Geometry: final body of the model. Coordinates: model frame, mm. A direction names the side the tool comes from. Coordinates: 2 decimals unless noted, no trailing zeros. Write each loop counter-clockwise with the first axis right and the second up, starting at its lowest first coordinate (ties: lowest second). Pieces come first, ordered by that corner, then holes.
Autodesk Inventor part; units mm, degrees
ref_plane "pc_body_XY" through (6, 12, 0) normal (1, 0, 0) x (0, 0, -1)
ref_plane "pc_body_YZ" through (6, 12, 0) normal (0, 0, -1) x (0, 1, 0)
ref_plane "pc_body_ZX" through (6, 12, 0) normal (0, 1, 0) x (1, 0, 0)
sketch "Sketch_1" plane through (0, 0, 0) normal (1, 0, 0) x (0, 1, 0)
  line L0 (16, 38.5) -> (0.5, 38.5)
  arc A0 (0.5, 38.5) -> (0, 38) centre (0.5, 38) ccw
  line L1 (0, 38) -> (0, 36.5)
  line L2 (0, 36.5) -> (15.75, 36.5)
  line L3 (15.75, 36.5) -> (15.75, 29.5)
  line L4 (15.75, 29.5) -> (12, 29.5)
  line L5 (12, 29.5) -> (12, 18.5)
  line L6 (12, 18.5) -> (15.75, 18.5)
  line L7 (15.75, 18.5) -> (15.75, -18.5)
  line L8 (15.75, -18.5) -> (12, -18.5)
  line L9 (12, -18.5) -> (12, -29.5)
  line L10 (12, -29.5) -> (15.75, -29.5)
  line L11 (15.75, -29.5) -> (15.75, -36.5)
  line L12 (15.75, -36.5) -> (0, -36.5)
  line L13 (0, -36.5) -> (0, -38)
  arc A1 (0, -38) -> (0.5, -38.5) centre (0.5, -38) ccw
  line L14 (0.5, -38.5) -> (16, -38.5)
  arc A2 (16, -38.5) -> (18, -36.5) centre (16, -36.5) ccw
  line L15 (18, -36.5) -> (18, 36.5)
  arc A3 (18, 36.5) -> (16, 38.5) centre (16, 36.5) ccw
extrude "Extrusion1" add sketch "Sketch_1" along normal blind 365
sketch "Sketch_3" plane through (6, 0, 0) normal (1, 0, 0) x (0, 0, -1)
  line L0 (-24, 19.95) -> (-24, 18)
  line L1 (-24, 18) -> (-27.8, 18)
  line L2 (-27.8, 18) -> (-27.8, 19.95)
  line L3 (-27.8, 19.95) -> (-24, 19.95)
  line L4 (-24, 19.95) -> (-24, 18)
revolve "Revolution1" add sketch "Sketch_3" angle 360 about axis through (6, 19.95, 24) along (0, 1, 0)
pattern_linear "Rectangular Pattern1" count 2 spacing 353.5 along (1, 0, 0) count 2 spacing 48 along (0, 0, -1) of "Revolution1"
ref_plane "pc_body_XY" through (6, 12, 0) normal (1, 0, 0) x (0, 0, -1)
ref_plane "pc_body_YZ" through (6, 12, 0) normal (0, 0, -1) x (0, 1, 0)
ref_plane "pc_body_ZX" through (6, 12, 0) normal (0, 1, 0) x (1, 0, 0)
properties part number "KR45H-340-Protected Cover"
Item 1: Section D-D, the plane x = 6. Output: boundary loops of the cut face in (y, z).
Derived:
outline: (0, -38) arc R0.5 ccw to (0.5, -38.5) - (16, -38.5) arc R2 ccw to (18, -36.5) - (18, -27.8) - (19.95, -27.8) - (19.95, -20.2) - (18, -20.2) - (18, 20.2) - (19.95, 20.2) - (19.95, 27.8) - (18, 27.8) - (18, 36.5) arc R2 ccw to (16, 38.5) - (0.5, 38.5) arc R0.5 ccw to (0, 38) - (0, 36.5) - (15.75, 36.5) - (15.75, 29.5) - (12, 29.5) - (12, 18.5) - (15.75, 18.5) - (15.75, -18.5) - (12, -18.5) - (12, -29.5) - (15.75, -29.5) - (15.75, -36.5) - (0, -36.5) - close
Item 2: Section C-C, the plane z = 24. Output: boundary loops of the cut face in (x, y).
Derived:
outline: (0, 12) - (365, 12) - (365, 18) - (363.3, 18) - (363.3, 19.95) - (355.7, 19.95) - (355.7, 18) - (9.8, 18) - (9.8, 19.95) - (2.2, 19.95) - (2.2, 18) - (0, 18) - close
Item 3: Section A-A, the plane y = 7. Output: boundary loops of the cut face in (x, z).
Derived:
outline: (0, -38.5) - (365, -38.5) - (365, -36.5) - (0, -36.5) - close; (0, 36.5) - (365, 36.5) - (365, 38.5) - (0, 38.5) - close
Item 4: Section B-B, the plane x = 88.5. Output: boundary loops of the cut face in (y, z), plus the area to 3 significant figures.
Derived:
outline: (0, -38) arc R0.5 ccw to (0.5, -38.5) - (16, -38.5) arc R2 ccw to (18, -36.5) - (18, 36.5) arc R2 ccw to (16, 38.5) - (0.5, 38.5) arc R0.5 ccw to (0, 38) - (0, 36.5) - (15.75, 36.5) - (15.75, 29.5) - (12, 29.5) - (12, 18.5) - (15.75, 18.5) - (15.75, -18.5) - (12, -18.5) - (12, -29.5) - (15.75, -29.5) - (15.75, -36.5) - (0, -36.5) - close
area: 317 mm2
Item 5: Material intervals for probe 1 along Z at (x, y) = (87, 15.5); probe 2 along Z at (x, y) = (62.5, 1.25); probe 3 along Y at (x, z) = (268.5, 21.5), sorted ascending.
Derived:
probe 1: z = -38.5 to -36.5, -29.5 to -18.5, 18.5 to 29.5, 36.5 to 38.5
probe 2: z = -38.5 to -36.5, 36.5 to 38.5
probe 3: y = 12 to 18
Item 6: Pull-direction query (Z, two-part tool) for faces 1 (the flat face through (180, 8, -38.5)), 2 (the flat face through (180, 8, 38.5)), 3 (the flat face through (360, 19.95, -24)), 4 (the flat face through (180, 12, -24)); classes: released by +Z, released by -Z, zero draft, split by the parting line, or undercut.
Derived:
face 1: released by -Z
face 2: released by +Z
face 3: zero draft
face 4: undercut
Item 7: Pin query (flat end, axial travel): pin 1 (3.5 mm diameter, centred on x = 146.5, z = -24, fed in from -Y); pin 2 (3.5 mm diameter, centred on x = 200, z = 32, fed in from -Y); pin 3 (6 mm diameter, centred on x = 248.5, z = 6.5, fed in from +Y). Return the tip coordinate at first contact, or that it passes through.
Derived:
pin 1: stops at y = 12
pin 2: stops at y = 15.75
pin 3: stops at y = 18
Item 8: Set-up query: faces 5 (the flat face through (180, 15.75, -33)), 6 (the cylindrical face through (7.141, 18.989, -20.375)), 7 (the flat face through (6, 19.95, -24)). Return all of +Z, -Z, +X, -X, +Y, -Y with unobstructed straight access to the full face (end or side cutting, diameter ignored); none if empty.
Derived:
face 5: +X, -X, -Y
face 6: +Y
face 7: +Z, -Z, +X, -X, +Y
